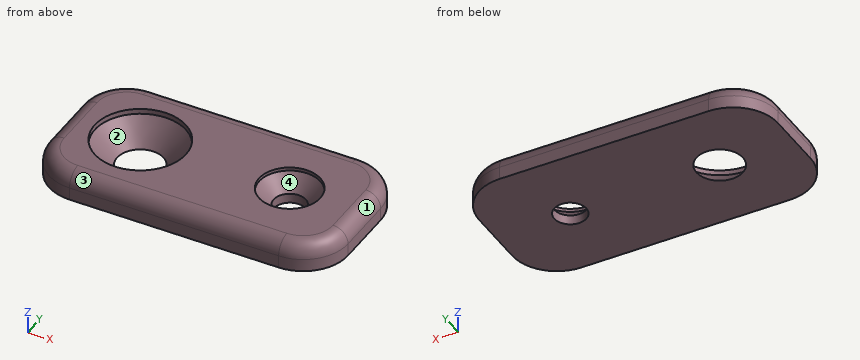
```python
from build123d import *

# Parameters (mm, degrees)
SKETCH1_W           = 40
SKETCH1_H           = 20
SKETCH1_R           = 3.1
SKETCH1_R_2         = 2.15
BOSS_EXTRUDE1_DEPTH = 3.7
SKETCH2_R           = 6.1
CUT_EXTRUDE1_DEPTH  = 0.7
CHAMFER1_SIZE       = 3
SKETCH3_R           = 4.1
CUT_EXTRUDE2_DEPTH  = 0.4
CHAMFER2_SIZE       = 2
FILLET1_R           = 6
FILLET2_R           = 2


# Some blends are built 0.0001 mm under size
with BuildPart() as part:
    # Sketch1 → Boss-Extrude1 (new body)
    with BuildSketch(Plane.XY):
        with Locations((10, 0)):
            Rectangle(SKETCH1_W, SKETCH1_H)
        Circle(SKETCH1_R, mode=Mode.SUBTRACT)
        with Locations((20, 0)):
            Circle(SKETCH1_R_2, mode=Mode.SUBTRACT)
    extrude(amount=BOSS_EXTRUDE1_DEPTH)

    # Sketch2 → Cut-Extrude1 (cut)
    with BuildSketch(Plane.XY.offset(3.7)):
        Circle(SKETCH2_R)
    extrude(amount=-CUT_EXTRUDE1_DEPTH, mode=Mode.SUBTRACT)

    # Chamfer1
    chamfer1_edges = [part.edges().sort_by_distance(p)[0] for p in [
        (-3.1, 0, 3),
    ]]
    chamfer(chamfer1_edges, length=CHAMFER1_SIZE - 0.0001)  # a hair under: the kernel refuses the full size

    # Sketch3 → Cut-Extrude2 (cut)
    with BuildSketch(Plane.XY.offset(3.7)):
        with Locations((20, 0)):
            Circle(SKETCH3_R)
    extrude(amount=-CUT_EXTRUDE2_DEPTH, mode=Mode.SUBTRACT)

    # Chamfer2
    # the kernel refuses this chamfer: 2 mm, written as the material it takes off along each edge
    with BuildSketch(Plane(origin=(20, 0, 3.3), x_dir=(1, 0, 0), z_dir=(0, 1, 0))) as chamfer2_piece_1_section:
        Polygon((2.15, CHAMFER2_SIZE), (2.15 + CHAMFER2_SIZE, 0), (2.15, 0), align=None)
    chamfer2_piece_1 = revolve(axis=Axis((20, 0, 3.3), (0, 0, -1)), mode=Mode.PRIVATE)
    chamfer2_piece_1 = chamfer2_piece_1 & Plane(origin=(20, 0, 2.270614155), x_dir=(1, 0, 0), z_dir=(0, 0, 1)) * Cylinder(4.1, 17, mode=Mode.PRIVATE)
    add(chamfer2_piece_1, mode=Mode.SUBTRACT)

    # Fillet1
    fillet1_edges = [part.edges().sort_by_distance(p)[0] for p in [
        (-10, 10, 1.85),
        (30, 10, 1.85),
        (30, -10, 1.85),
        (-10, -10, 1.85),
    ]]
    fillet(fillet1_edges, radius=FILLET1_R)

    # Fillet2
    fillet2_edges = [part.edges().sort_by_distance(p)[0] for p in [
        (30, 0, 3.7),
        (10, -10, 3.7),
        (-10, 0, 3.7),
        (10, 10, 3.7),
        (-8.242640687, 8.242640687, 3.7),
        (28.242640687, 8.242640687, 3.7),
        (-8.242640687, -8.242640687, 3.7),
        (28.242640687, -8.242640687, 3.7),
    ]]
    fillet(fillet2_edges, radius=FILLET2_R)


solid = part.part
```
Here's how the part is built. I have some questions about the finished solid (model axes, mm). Face numbers are marked on the shaded views. Give positions to 0.01 mm unless a question says otherwise; leave off trailing zeros. Loops run counter-clockwise (first coordinate to the right, second up) from the corner with the lowest first, then second, coordinate; pieces in that order, holes last. Notation, with made-up numbers: M 62,-38.75 L 104,-38.75 A34 ccw 104,-6.75 Z; hole C 20.25,-26.5 d10. An arc over 180 degrees is marked long. Return JSON: item names as keys, results as strings.
Item 1: Imagine slicing it at D-D on x = 20. List the corners of the cut face in (y, z) for me.
A:
{"outline": "M -10,0 L -2.15,0 L -2.15,1.3 L -4.1,3.25 L -4.1,3.7 L -8,3.7 A2 ccw -10,1.7 Z; M 2.15,0 L 10,0 L 10,1.7 A2 ccw 8,3.7 L 4.1,3.7 L 4.1,3.25 L 2.15,1.3 Z"}
Item 2: Thinking about a two-plate mould opening in Y: for the marked faces 1, 2, 3 and 4, which applies, released by +Y, released by -Y, zero draft, split by the parting line, or undercut?
A:
{"face 1": "zero draft", "face 2": "undercut", "face 3": "released by -Y", "face 4": "undercut"}
Item 3: Please list where these lines run through material, in increasing order: line 1 (X direction, y = 0, z = 0.05); line 2 (X direction, y = 0.5, z = 0.25); line 3 (Y direction, x = 20, z = 0.5).
A:
{"line 1": "x = -10 to -3.15, 3.15 to 17.85, 22.15 to 30", "line 2": "x = -10 to -3.31, 3.31 to 17.91, 22.09 to 30", "line 3": "y = -10 to -2.15, 2.15 to 10"}
Item 4: Imagine slicing it at B-B on y = 0. State how many separate pieces and enclosed holes the cut face has, then the cut area to 3 significant figures.
A:
{"separate pieces": "3", "enclosed holes": "0", "area": "88.7 mm^2"}
Item 5: I'm going to push flat-ended pins straight in: pin 1 Ø2 at (x, z) = (-5.5, 2.5) entering from -Y; pin 2 Ø1.5 at (y, z) = (4.5, 2) entering from -X; pin 3 Ø7.5 at (x, y) = (0, 0) entering from +Z. Where does each tip first touch, or does it pass through?
A:
{"pin 1": "stops at y = -9.95", "pin 2": "stops at x = -10", "pin 3": "stops at z = 0.65"}
Item 6: Imagine slicing it at C-C on z = 2.45. List the corners of the cut face in (x, y) for me, then the cut area to 3 significant figures.
A:
{"outline": "M -9.85,-4 A5.85 ccw -4,-9.85 L 24,-9.85 A5.85 ccw 29.85,-4 L 29.85,4 A5.85 ccw 24,9.85 L -4,9.85 A5.85 ccw -9.85,4 Z; hole C 0,0 d11.1; hole C 20,0 d6.6", "area": "622 mm^2"}
